from build123d import *

# Parameters (mm, degrees)
BOSS_EXTRUDE1_DEPTH = 3.175
SKETCH7_R           = 3.2639
CUT_EXTRUDE3_DEPTH  = 678.24348403


with BuildPart() as part:
    # Sketch2 → Boss-Extrude1 (new body)
    with BuildSketch(Plane(origin=(-112.555, 0, -573.58969557), x_dir=(0, 0.6231241879767124, 0.7821229100073485), z_dir=(-1, 0, 0))):
        with BuildLine():
            Line((843.785187932, 138.582376841), (864.330586832, 122.213677187))
            ThreePointArc((864.330586832, 122.213677187), (874.263547789, 127), (884.196508746, 122.213677187))
            Line((884.196508746, 122.213677187), (887.645495372, 124.961515108))
            ThreePointArc((887.645495372, 124.961515108), (888.526447304, 126.330171585), (888.395706135, 127.952578317))
            Line((888.395706135, 127.952578317), (869.77401473, 171.202610873))
            Line((869.77401473, 171.202610873), (862.593047153, 162.189320479))
            Line((862.593047153, 162.189320479), (875.624929298, 131.921966414))
            add(Edge.make_bspline(
                [(866.008867214, 133.866862107), (871.18323177, 134.685144315), (875.624929298, 131.921966414)],
                knots=[0, 0, 0, 1, 1, 1], degree=2))
            Line((866.008867214, 133.866862107), (850.116129682, 146.528745607))
            Line((850.116129682, 146.528745607), (843.785187932, 138.582376841))
        make_face()
    extrude(amount=BOSS_EXTRUDE1_DEPTH)

    # Sketch7 → Cut-Extrude3 (cut, through all)
    with BuildSketch(Plane.ZY.offset(115.73)):
        with Locations((5.08, 639.251411908)):
            Circle(SKETCH7_R)
        with Locations((5.08, 667.397263635)):
            Circle(SKETCH7_R)
    extrude(amount=-CUT_EXTRUDE3_DEPTH, mode=Mode.SUBTRACT)


solid = part.part
Could you check a few things on this model? Use its own coordinates, in mm. A direction names the side the tool comes from. Give positions to 0.01 mm unless a question says otherwise; leave off trailing zeros. Order: outer loops, then holes, each group sorted by start corner. A loop starts at its lowest first (then second) coordinate and runs counter-clockwise, first axis right, second up.
1. Suppose I cut it at D-D (x = -114.4). Give the number of separate pieces and of enclosed holes in the cut face, plus the area to 3 significant figures.
2. For faces 1 (the flat face through (-114.12, 664.61, 21.05)), 2 (the flat face through (-114.1, 656.7, 14.3)), which set-ups out of +Z, -Z, +X, -X, +Y, -Y let a thin tool reach every point of the face, with its end or its side?
3. Suppose I cut it at C-C (z = 10.5). List the corners of the cut face in (x, y) for me (3 decimals), plus the area to 3 significant figures.
4. We'd pull the mould along Z, two halves only. Please class faces 3 (the cylindrical face through (-114.12, 644.004, 30.931)), 4 (the flat face through (-114, 634.171, 13)), 5 (the flat face through (-114.1, 648.7, 42.3)): pulls with the +Z half, pulls with the -Z half, needs draft (parallel to the pull), parting line crosses it, or undercut.
5. Will these pins go through, and if not, where does the flat tip stop? P1, Ø1.5, axis at y = 649, z = 25.5, coming from the +X side; P2, Ø1, axis at x = -113.5, z = 7, coming from the +Y side.
6. Suppose I cut it at B-B (z = 5.08). List the corners of the cut face in (x, y) for me (3 decimals), plus the area to 3 significant figures.
7. Suppose I cut it at A-A (y = 642). List the corners of the cut face in (x, z) for me (3 decimals), plus the area to 3 significant figures.
8. I need wall thicknesses on L1, parallel to Y at x = -114.4, z = 5.08; L2, parallel to Z at x = -113.5, y = 668; L3, parallel to Y at x = -114.7, z = 17. Which ranges of each line are inside material? Lowest first, please.
Solved:
1. separate pieces: 1
1. enclosed holes: 2
1. area: 720 mm2
2. face 1: +Z, +X, -X, +Y
2. face 2: -Z, +X, -X
3. outline: (-115.73, 634.171) - (-112.555, 634.171) - (-112.555, 644.331) - (-115.73, 644.331) - close; (-115.73, 658.734) - (-112.555, 658.734) - (-112.555, 670.258) - (-115.73, 670.258) - close
3. area: 68.8 mm2
4. face 3: undercut
4. face 4: needs draft
4. face 5: pulls with the +Z half
5. P1: passes through
5. P2: stops at y = 672.4
6. outline: (-115.73, 634.171) - (-112.555, 634.171) - (-112.555, 635.988) - (-115.73, 635.988) - close; (-115.73, 642.515) - (-112.555, 642.515) - (-112.555, 644.331) - (-115.73, 644.331) - close; (-115.73, 661.635) - (-112.555, 661.635) - (-112.555, 664.133) - (-115.73, 664.133) - close; (-115.73, 670.661) - (-112.555, 670.661) - (-112.555, 673.159) - (-115.73, 673.159) - close
6. area: 27.4 mm2
7. outline: (-115.73, 0) - (-112.555, 0) - (-112.555, 3.32) - (-115.73, 3.32) - close; (-115.73, 6.84) - (-112.555, 6.84) - (-112.555, 28.969) - (-115.73, 28.969) - close
7. area: 80.8 mm2
8. L1: y = 634.17 to 635.99, 642.52 to 644.33, 661.64 to 664.13, 670.66 to 673.16
8. L2: z = 0 to 1.87, 8.29 to 14.72
8. L3: y = 634.17 to 644.33, 655.25 to 666.78
